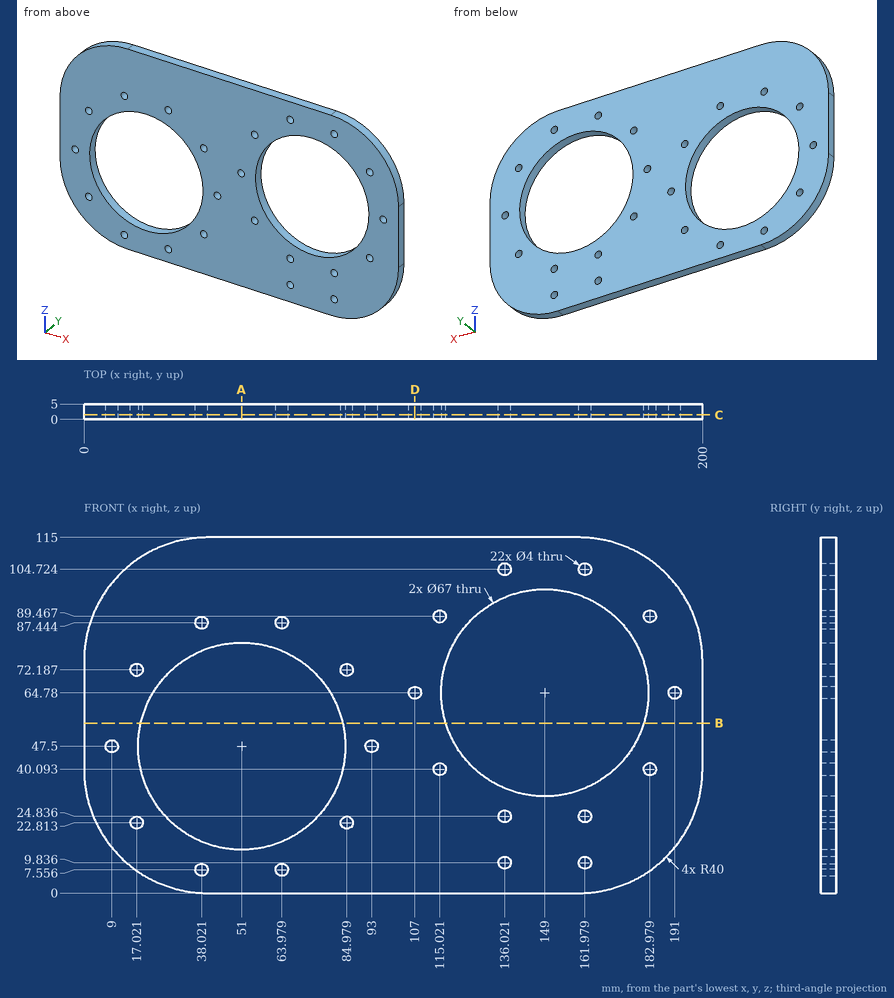
The figure shows three views and two pictorial views of one solid part (mm, origin at its lowest corner). Answer the questions. Coordinates: 2 decimals unless noted, no trailing zeros. Order: outer loops, then holes, each group sorted by start corner. A loop starts at its lowest first (then second) coordinate and runs counter-clockwise, first axis right, second up.
Q1. Consider line 1 (X direction, y = 1.7, z = 77.5) (1 decimal); line 2 (X direction, y = 0.25, z = 106); line 3 (Z direction, x = 49.5, y = 2.7). Determine where each line is inside the solid, lowest interval first.
Q2. A cutting plane is placed at A-A, the plane x = 51. Write down the section's boundary in (y, z).
Q3. A cutting plane is placed at C-C, the plane y = 1.5. State how many separate pieces and enclosed holes the cut face has, and give its area (3 significant figures).
Q4. A cutting plane is placed at D-D, the plane x = 107. Write down the section's boundary in (y, z), and give its area (3 significant figures).
Q5. A cutting plane is placed at B-B, the plane z = 55. Write down the section's boundary in (x, y).
Q6. Given P1, Ø2.5, axis at x = 182.98, z = 89.47, coming from the -Y side; P2, Ø1.5, axis at x = 25, y = 3.5, coming from the -Z side (1 decimal), each flat-ended and moving along its own axis, determine where each tip first touches the part or whether it passes through.
Answers follow:
1. line 1: x = 0.1 to 36.1, 65.9 to 118, 180 to 199.9
1. line 2: x = 14.72 to 134.48, 137.56 to 160.44, 163.52 to 185.28
1. line 3: z = 0 to 14.03, 80.97 to 115
2. outline: (0, 0) - (5, 0) - (5, 14) - (0, 14) - close; (0, 81) - (5, 81) - (5, 115) - (0, 115) - close
3. separate pieces: 1
3. enclosed holes: 24
3. area: 14,300 mm2
4. outline: (0, 0) - (5, 0) - (5, 62.78) - (0, 62.78) - close; (0, 66.78) - (5, 66.78) - (5, 115) - (0, 115) - close
4. area: 555 mm2
5. outline: (0, 0) - (18.35, 0) - (18.35, 5) - (0, 5) - close; (83.65, 0) - (116.96, 0) - (116.96, 5) - (83.65, 5) - close; (181.04, 0) - (200, 0) - (200, 5) - (181.04, 5) - close
6. P1: passes through
6. P2: stops at z = 2.6
